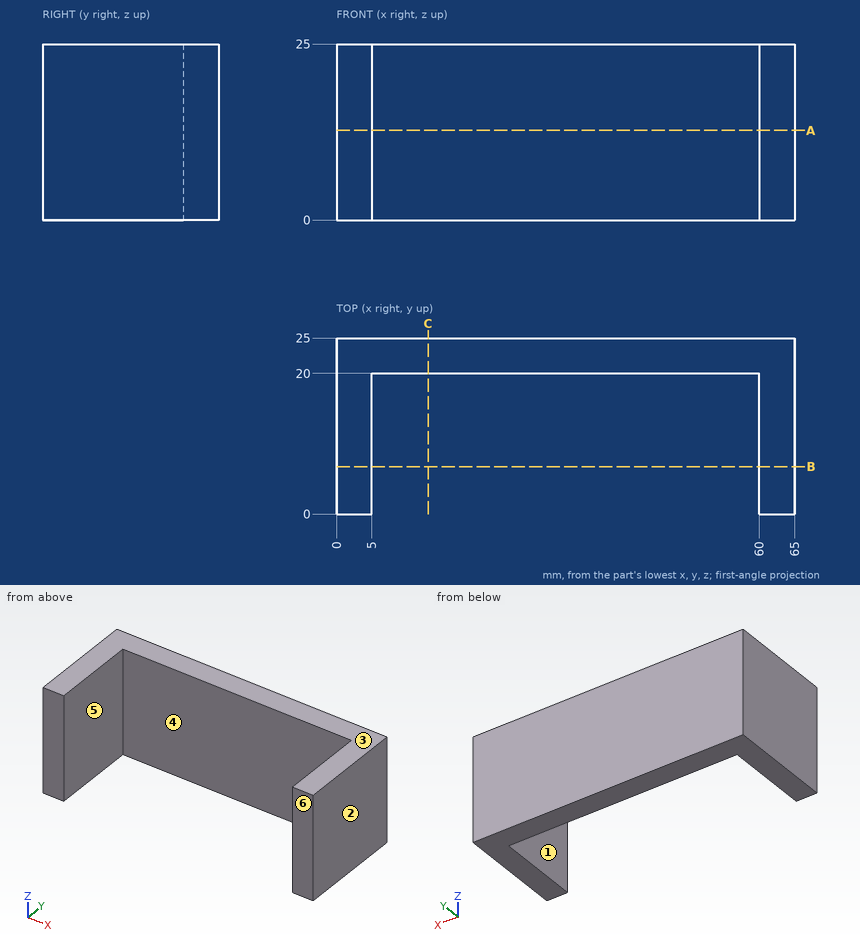
The drawing under review shows one solid part. Ordinate dimensions are in mm from its lowest x, y, z. A direction names the side the tool comes from. Give positions to 0.01 mm unless a question says otherwise; leave off trailing zeros. Loops run counter-clockwise (first coordinate to the right, second up) from the corner with the lowest first, then second, coordinate; pieces in that order, holes last. Notation, with made-up numbers: M 48,4 L 56,4 A17 ccw 56,27 Z; hole C -21.5,-15 d8. An arc over 180 degrees is marked long. One line per item, written item: value. Start each with the question number.
Q1. Clearance check with a flat-ended pin moving along its axis: pin 1 Ø1 at (x, z) = (43.5, 16) entering from -Y. State where the tip first meets the part, or that it passes through.
Q2. Draft analysis for pull direction X (two halves, no side actions). For the marked faces 1, 2, 3 and 4, state which applies: released by +X, released by -X, zero draft, split by the parting line, or undercut.
Q3. Add section B-B (y = 6.75). Give the boundary of the cut face in (x, z).
Q4. Add section A-A (z = 12.75). Give the boundary of the cut face in (x, y).
Q5. Add section C-C (x = 13). Give the boundary of the cut face in (y, z), and give its area (3 significant figures).
Q6. For L1, parallel to X at y = 3.75, z = 20.5; L2, parallel to Y at x = 9, z = 20.5, list the stretches that pass through material, from the lowest coordinate up.
Q7. Machinability: for the marked faces 5 and 6, which of the approach directions +Z, -Z, +X, -X, +Y, -Y give a long, thin tool a straight path to every point of the face, cutting with its end or side? Answer none if there is none.
Reply:
1. pin 1: y = 20
2. face 1: undercut
2. face 2: released by +X
2. face 3: zero draft
2. face 4: undercut
3. outline: M 0,0 L 5,0 L 5,25 L 0,25 Z; M 60,0 L 65,0 L 65,25 L 60,25 Z
4. outline: M 0,0 L 5,0 L 5,20 L 60,20 L 60,0 L 65,0 L 65,25 L 0,25 Z
5. outline: M 20,0 L 25,0 L 25,25 L 20,25 Z
5. area: 125 mm²
6. L1: 0 to 5, 60 to 65
6. L2: 20 to 25
7. face 5: +Z, -Z, -Y
7. face 6: +Z, -Z, +X, -X, -Y
